from build123d import *

# Parameters (mm, degrees)
SKETCH1_R           = 6
SKETCH1_R_2         = 1.7
BOSS_EXTRUDE1_DEPTH = 2
CHAMFER1_SIZE       = 1.5
SKETCH2_R           = 6
SKETCH2_R_2         = 1.5
BOSS_EXTRUDE2_DEPTH = 2
CHAMFER2_SIZE       = 1.5


with BuildPart() as part:
    # Sketch1 → Boss-Extrude1 (new body)
    with BuildSketch(Plane.XY):
        Circle(SKETCH1_R)
        Circle(SKETCH1_R_2, mode=Mode.SUBTRACT)
    extrude(amount=BOSS_EXTRUDE1_DEPTH)

    # Chamfer1
    chamfer1_edges = [part.edges().sort_by_distance(p)[0] for p in [
        (-6, 0, 2),
    ]]
    chamfer(chamfer1_edges, length=CHAMFER1_SIZE)

    # Sketch2 → Boss-Extrude2 (add)
    with BuildSketch(Plane.XY.offset(2)):
        Circle(SKETCH2_R)
        Circle(SKETCH2_R_2, mode=Mode.SUBTRACT)
    extrude(amount=BOSS_EXTRUDE2_DEPTH)

    # Chamfer2
    chamfer2_edges = [part.edges().sort_by_distance(p)[0] for p in [
        (-6, 0, 2),
    ]]
    chamfer(chamfer2_edges, length=CHAMFER2_SIZE - 0.0001)  # a hair under: the kernel refuses the full size


solid = part.part
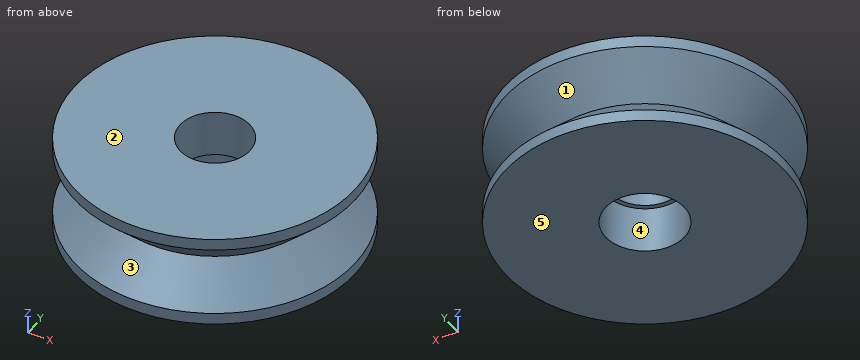
Build history of the part. All positions in model axes, mm. Face numbers are marked on the shaded views. A direction names the side the tool comes from. Round coordinates to 2 decimals unless told otherwise and drop trailing zeros. Order: outer loops, then holes, each group sorted by start corner. A loop starts at its lowest first (then second) coordinate and runs counter-clockwise, first axis right, second up. Notation, with made-up numbers: M -35,-5 L 4,-5 A5 cw 4,2 Z; hole C -7.5,-0.75 d8. An arc over 180 degrees is marked long. Use CSV: the item, a comma, the result in double quotes. Start each with the question number.
(1) Flat gauge pins, fed straight in: P1, Ø1.5, axis at y = 3.5, z = 1.5, coming from the +X side; P2, Ø1.5, axis at y = 1, z = 2, coming from the -X side. Where does each tip first touch, or does it go through?
(2) Drill centre lines: probe 1 along Y at (x, z) = (0, 0.7); probe 2 along Y at (x, z) = (0, 0.8); probe 3 along Z at (x, y) = (2.75, 5). Where is each one in solid material? Low to high.
(3) Tool access for the marked faces 1 and 2: list every direction of +Z, -Z, +X, -X, +Y, -Y with a clear straight run to the whole face (end or side of a thin tool).
(4) Cut at C-C on z = 1.85. List the corners of the cut face in (x, y).
(5) Mould opens along Z. For the marked faces 3, 4 and 5 say: +Z half, -Z half, draft (parallel to the pull), parting line (faces both ways), or undercut.
(6) Cut at D-D on z = 0.8. List the corners of the cut face in (x, y), then the cut area to 3 significant figures.
Findings:
1,P1,"stops at x = 4.71"
1,P2,"stops at x = -5.17"
2,probe 1,"y = -5.8 to -1.7, 1.7 to 5.8"
2,probe 2,"y = -5.7 to -1.7, 1.7 to 5.7"
2,probe 3,"z = 0 to 0.79, 3.21 to 4"
3,face 1,"none"
3,face 2,"+Z, +X, -X, +Y, -Y"
4,outline,"C 0,0 d9.3; hole C 0,0 d3.4"
5,face 3,"undercut"
5,face 4,"draft"
5,face 5,"-Z half"
6,outline,"C 0,0 d11.4; hole C 0,0 d3.4"
6,area,"93.0 mm^2"
